from build123d import *

# Parameters (mm, degrees)
SKETCH1_R           = 11
SKETCH1_R_2         = 4
BOSS_EXTRUDE1_DEPTH = 7
SKETCH2_R           = 9.5
SKETCH2_R_2         = 5.5
CUT_EXTRUDE1_DEPTH  = 1
SKETCH3_R           = 9.5
SKETCH3_R_2         = 5.5
CUT_EXTRUDE2_DEPTH  = 1


with BuildPart() as part:
    # Sketch1 → Boss-Extrude1 (new body)
    with BuildSketch(Plane.XY):
        Circle(SKETCH1_R)
        Circle(SKETCH1_R_2, mode=Mode.SUBTRACT)
    extrude(amount=BOSS_EXTRUDE1_DEPTH)

    # Sketch2 → Cut-Extrude1 (cut)
    with BuildSketch(Plane.XY.offset(7)):
        Circle(SKETCH2_R)
        Circle(SKETCH2_R_2, mode=Mode.SUBTRACT)
    extrude(amount=-CUT_EXTRUDE1_DEPTH, mode=Mode.SUBTRACT)

    # Sketch3 → Cut-Extrude2 (cut)
    with BuildSketch(Plane(origin=(0, 0, 0), x_dir=(-1, 0, 0), z_dir=(0, 0, -1))):
        Circle(SKETCH3_R)
        Circle(SKETCH3_R_2, mode=Mode.SUBTRACT)
    extrude(amount=-CUT_EXTRUDE2_DEPTH, mode=Mode.SUBTRACT)


solid = part.part
The model under review builds one solid part; all positions refer to its coordinate system, in mm. A direction names the side the tool comes from. Round coordinates to 2 decimals unless told otherwise and drop trailing zeros. Loops run counter-clockwise (first coordinate to the right, second up) from the corner with the lowest first, then second, coordinate; pieces in that order, holes last. Notation, with made-up numbers: M -28,68 L 25,68 A22 ccw 25,103 Z; hole C 53,3 d5. An arc over 180 degrees is marked long. Answer as a JSON object with one key per item and string values.
Item 1: For line 1 along Y through (x, z) = (0, 6.8); line 2 along Y through (x, z) = (0, 5.25); line 3 along X through (y, z) = (3.5, 6.5), list the stretches that pass through material, from the lowest coordinate up.
Check sheet entries:
{"line 1": "-11 to -9.5, -5.5 to -4, 4 to 5.5, 9.5 to 11", "line 2": "-11 to -4, 4 to 11", "line 3": "-10.43 to -8.83, -4.24 to -1.94, 1.94 to 4.24, 8.83 to 10.43"}
Item 2: We need section A-A, the plane y = 0. State the section outline as (x, z) points.
Check sheet entries:
{"outline": "M -11,0 L -9.5,0 L -9.5,1 L -5.5,1 L -5.5,0 L -4,0 L -4,7 L -5.5,7 L -5.5,6 L -9.5,6 L -9.5,7 L -11,7 Z; M 4,0 L 5.5,0 L 5.5,1 L 9.5,1 L 9.5,0 L 11,0 L 11,7 L 9.5,7 L 9.5,6 L 5.5,6 L 5.5,7 L 4,7 Z"}
Item 3: We need section D-D, the plane x = -6. State the section outline as (y, z) points.
Check sheet entries:
{"outline": "M -9.22,0 L -7.37,0 L -7.37,1 L 7.37,1 L 7.37,0 L 9.22,0 L 9.22,7 L 7.37,7 L 7.37,6 L -7.37,6 L -7.37,7 L -9.22,7 Z"}
Item 4: The part is to be moulded in two halves that separate along Y. For faces 1 (the face through (-4, -2, 7)), 2 (the face through (-0.867, -3.905, 3.451)), 3 (the face through (-2.38, -10.74, 3.45)), say which applies: +Y half, -Y half, draft (parallel to the pull), parting line (faces both ways), or undercut.
Check sheet entries:
{"face 1": "draft", "face 2": "undercut", "face 3": "parting line"}
Item 5: Tool access review of faces 4 (the face through (-10, 0, 7)), 5 (the face through (-1.19, -5.37, 6.51)), 6 (the face through (-4, -4, 1)): name each direction out of +Z, -Z, +X, -X, +Y, -Y from which nothing blocks a thin tool from reaching the whole face with its end or side.
Check sheet entries:
{"face 4": "+Z, +X, -X, +Y, -Y", "face 5": "+Z", "face 6": "-Z"}
Item 6: We need section C-C, the plane z = 5.5. State the section outline as (x, y) points, and give its area (3 significant figures).
Check sheet entries:
{"outline": "C 0,0 d22; hole C 0,0 d8", "area": "330 mm2"}
Item 7: Clearance check with flat-ended pins moving along their axes: P1, Ø2, axis at x = -4.5, z = 2.5, coming from the -Y side; P2, Ø3, axis at y = 8.5, z = 2, coming from the -X side; P3, Ø6, axis at x = -5, y = 2.5, coming from the -Z side; P4, Ø4, axis at y = -8.5, z = 3.5, coming from the -X side. State where each tip first meets the part, or that it passes through.
Check sheet entries:
{"P1": "y = -10.43", "P2": "x = -8.49", "P3": "z = 0", "P4": "x = -8.87"}
